```python
from build123d import *

# Parameters (mm, degrees)
F0_W     = 6.35
F0_H     = 190.5
F1_DEPTH = 38.35
F0_W_2   = 22
F0_R     = 5
F2_DEPTH = 6.35
F3_W     = 55
F3_H     = 70
F4_DEPTH = 6.35


with BuildPart() as f1:
    # F0 (on Front) → F1 (new body)
    with BuildSketch(Plane.XZ):
        with Locations((49.325, 95.25)):
            Rectangle(F0_W, F0_H)
        with Locations((77.675, 95.25)):
            Rectangle(F0_W, F0_H)
    extrude(amount=F1_DEPTH)

    # F0 (on Front) → F2 (join)
    with BuildSketch(Plane.XZ):
        Polygon((0, 25.1), (0, 0), (46.15, 0), (46.15, 190.5), (0, 190.5), (0, 158.75), (19.05, 158.75), (19.05, 31.45), (0, 31.45), align=None)
        with Locations((49.325, 95.25)):
            Rectangle(F0_W, F0_H)
        with Locations((63.5, 95.25)):
            Rectangle(F0_W_2, F0_H)
        with Locations((63.5, 20)):
            Circle(F0_R, mode=Mode.SUBTRACT)
        with Locations((77.675, 95.25)):
            Rectangle(F0_W, F0_H)
        Polygon((80.85, 190.5), (80.85, 0), (127, 0), (127, 31.45), (107.95, 31.45), (107.95, 158.75), (127, 158.75), (127, 190.5), align=None)
    extrude(amount=F2_DEPTH)

    # F3 (on face) → F4 (join)
    with BuildSketch(Plane.XZ.offset(38.35)):
        with Locations((63.5, 155.5)):
            Rectangle(F3_W, F3_H)
    extrude(amount=F4_DEPTH)


solid = f1.part
```
Check sheet for the modelled part. Datum: model origin and axes. Units: mm. A direction names the side the tool comes from. Give positions to 0.01 mm unless a question says otherwise; leave off trailing zeros. Write each loop counter-clockwise with the first axis right and the second up, starting at its lowest first coordinate (ties: lowest second). Pieces come first, ordered by that corner, then holes. Notation, with made-up numbers: (-18.75, 24.25) -> (27.25, 24.25) arc R24 ccw to (27.25, 54.25) -> close; hole circle Ø1 at (73.25, 7). An arc over 180 degrees is marked (long way). Use CSV: the item, a comma, the result in double quotes. Start each with the question number.
Q1. Cross-section at C-C on z = 101.5. Enter the section's corners in (x, y), and give its area (3 significant figures).
Q2. Tool access check on faces 1 (the flat face through (86, -38.35, 156)), 2 (the flat face through (41, -38.35, 156)), 3 (the flat face through (19.05, -3, 96)), 4 (the flat face through (36, -41, 155)), 5 (the flat face through (107.95, -3, 94)). Record the directions out of +Z, -Z, +X, -X, +Y, -Y that give a thin tool (end or side, any length) a straight path to the whole face; none if there is none.
Q3. Depth check by flat-ended pin: P1, Ø4, axis at y = -35.5, z = 46, coming from the -X side; P2, Ø7, axis at x = 48.5, z = 72, coming from the -Y side; P3, Ø5, axis at y = -3.5, z = 122, coming from the +X side; P4, Ø1.5, axis at x = 17.5, z = 70, coming from the +Y side. Enter the tip coordinate at first touch or a pass-through.
Q4. Scan lines: line 1 along Z through (x, y) = (63.5, -1.5); line 2 along X through (y, z) = (-36, 122.5); line 3 along Y through (x, z) = (55.5, 129.5). Record each from-to range of solid material in increasing order.
Q5. Cross-section at B-B on x = 63.5. Enter the section's corners in (y, z).
Q6. Cross-section at A-A on y = -12.5. Enter the section's corners in (x, z), and give its area (3 significant figures).
Q7. Cross-section at D-D on z = 20. Enter the section's corners in (x, y), and give its area (3 significant figures).
Q8. Release check for a two-part mould opening along X. For faces 6 (the flat face through (74.5, -22, 94)), 7 (the flat face through (0, -3, 175)), 8 (the cylindrical face through (62.42, -3.13, 15.12)), 9 (the flat face through (63, -44.7, 156)) record: +X half, -X half, draft (parallel to the pull), parting line (faces both ways), or undercut.
Working result:
1,outline,"(19.05, -6.35) -> (46.15, -6.35) -> (46.15, -38.35) -> (52.5, -38.35) -> (52.5, -6.35) -> (74.5, -6.35) -> (74.5, -38.35) -> (80.85, -38.35) -> (80.85, -6.35) -> (107.95, -6.35) -> (107.95, 0) -> (19.05, 0) -> close"
1,area,"971 mm^2"
2,face 1,"+Z, -Z, +X"
2,face 2,"+Z, -Z, -X"
2,face 3,"-X, +Y, -Y"
2,face 4,"+Z, -Z, -X, -Y"
2,face 5,"+X, +Y, -Y"
3,P1,"stops at x = 46.15"
3,P2,"stops at y = -38.35"
3,P3,"stops at x = 107.95"
3,P4,"passes through"
4,line 1,"z = 0 to 15, 25 to 190.5"
4,line 2,"x = 46.15 to 52.5, 74.5 to 80.85"
4,line 3,"y = -44.7 to -38.35, -6.35 to 0"
5,outline,"(-44.7, 120.5) -> (-38.35, 120.5) -> (-38.35, 190.5) -> (-44.7, 190.5) -> close; (-6.35, 0) -> (0, 0) -> (0, 15) -> (-6.35, 15) -> close; (-6.35, 25) -> (0, 25) -> (0, 190.5) -> (-6.35, 190.5) -> close"
6,outline,"(46.15, 0) -> (52.5, 0) -> (52.5, 190.5) -> (46.15, 190.5) -> close; (74.5, 0) -> (80.85, 0) -> (80.85, 190.5) -> (74.5, 190.5) -> close"
6,area,"2,420 mm^2"
7,outline,"(0, -6.35) -> (46.15, -6.35) -> (46.15, -38.35) -> (52.5, -38.35) -> (52.5, -6.35) -> (58.5, -6.35) -> (58.5, 0) -> (0, 0) -> close; (68.5, -6.35) -> (74.5, -6.35) -> (74.5, -38.35) -> (80.85, -38.35) -> (80.85, -6.35) -> (127, -6.35) -> (127, 0) -> (68.5, 0) -> close"
7,area,"1,150 mm^2"
8,face 6,"undercut"
8,face 7,"-X half"
8,face 8,"undercut"
8,face 9,"draft"
